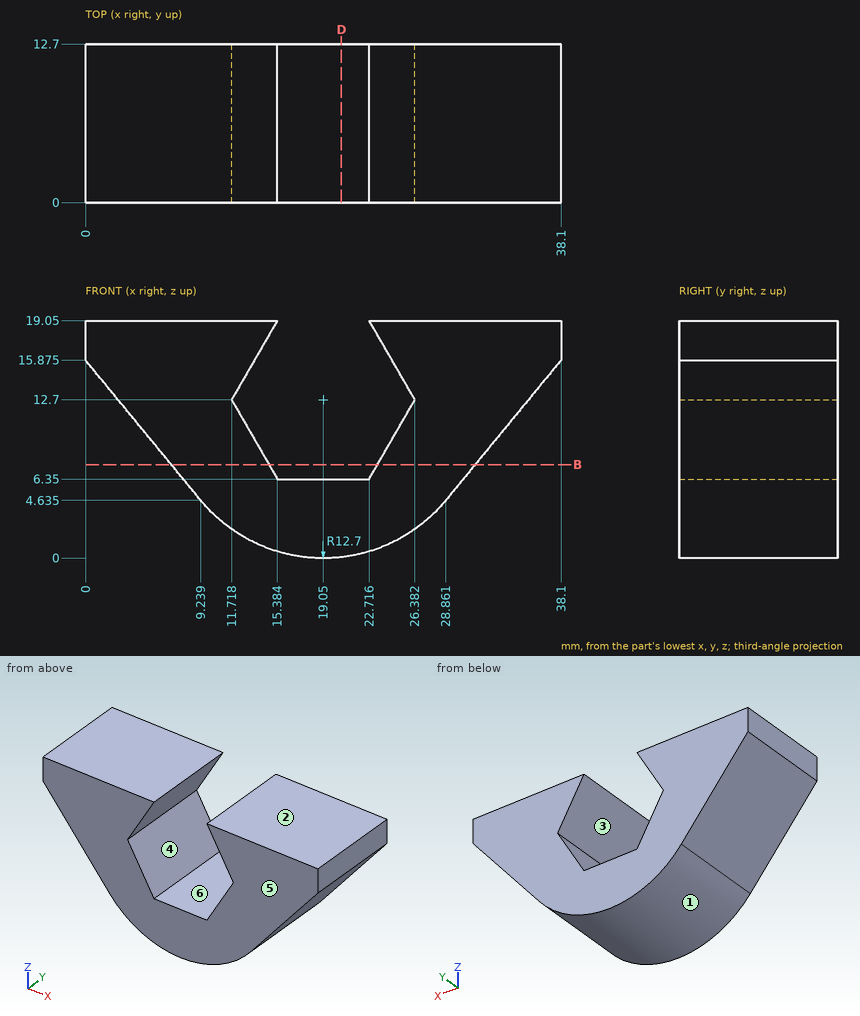
The drawing under review shows one solid part. Ordinate dimensions are in mm from its lowest x, y, z. A direction names the side the tool comes from. Coordinates: 2 decimals unless noted, no trailing zeros. Order: outer loops, then holes, each group sorted by start corner. A loop starts at its lowest first (then second) coordinate and runs counter-clockwise, first axis right, second up. Notation, with made-up numbers: (-30.5, 29) -> (10.5, 29) arc R22 cw to (10.5, 65) -> close; hole circle Ø3 at (80.5, 10.25). An arc over 180 degrees is marked (long way). Answer as CSV lines item,"result".
Q1. For the marked faces 5 and 6, list the 3-axis set-ups (+Z, -Z, +X, -X, +Y, -Y) from which the entire face can be reached by the end or side of a thin tool; tool diameter is ignored.
Model answer:
face 5,"+Z, -Z, +X, -X, -Y"
face 6,"+Z, +Y, -Y"
Q2. We need section D-D (x = 20.5). State the section outline as (y, z) points.
Model answer:
outline,"(0, 0.08) -> (12.7, 0.08) -> (12.7, 6.35) -> (0, 6.35) -> close"
Q3. Draft analysis for pull direction X (two halves, no side actions). For the marked faces 1, 2, 3 and 4, state which applies: released by +X, released by -X, zero draft, split by the parting line, or undercut.
Model answer:
face 1,"split by the parting line"
face 2,"zero draft"
face 3,"undercut"
face 4,"undercut"
Q4. Clearance check with flat-ended pins moving along their axes: pin 1 Ø5 at (x, y) = (28, 4) entering from -Z; pin 2 Ø4 at (y, z) = (9, 5) entering from +X (1 decimal); pin 3 Ø8 at (x, z) = (14, 13.5) entering from -Y; pin 4 Ø6 at (x, y) = (19, 6) entering from +Z. State where each tip first meets the part, or that it passes through.
Model answer:
pin 1,"stops at z = 1.76"
pin 2,"stops at x = 30.8"
pin 3,"stops at y = 0"
pin 4,"stops at z = 6.35"
Q5. We need section B-B (z = 7.5). State the section outline as (x, y) points (1 decimal), plus the area to 3 significant figures.
Model answer:
outline,"(6.9, 0) -> (14.7, 0) -> (14.7, 12.7) -> (6.9, 12.7) -> close; (23.4, 0) -> (31.2, 0) -> (31.2, 12.7) -> (23.4, 12.7) -> close"
area,"199 mm2"
Q6. Wall thickness on line 1 along X through (y, z) = (10, 10.75) (1 decimal); line 2 along X through (y, z) = (7.5, 18.75); line 3 along X through (y, z) = (11, 3.5) (1 decimal): over which ranges is each line inside the solid? List them lowest first. Write a range as [from, to].
Model answer:
line 1,"x = [4.2, 12.8], [25.3, 33.9]"
line 2,"x = [0, 15.21], [22.89, 38.1]"
line 3,"x = [10.3, 27.8]"
